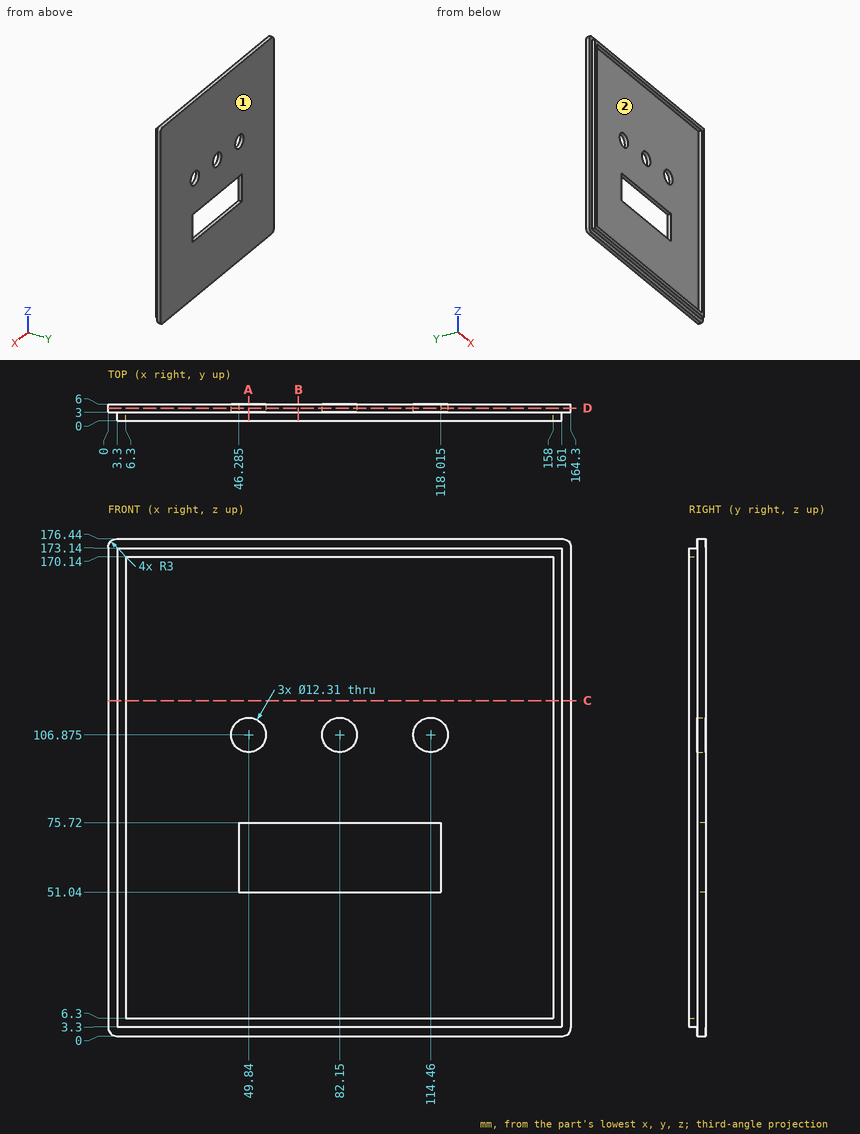
Job drawing, mm, ordinate dimensions from the low corner. One solid piece. Round coordinates to 2 decimals unless told otherwise and drop trailing zeros. Write each loop counter-clockwise with the first axis right and the second up, starting at its lowest first coordinate (ties: lowest second). Pieces come first, ordered by that corner, then holes. Notation, with made-up numbers: M 81.25,36 L 93.25,36 A31 ccw 93.25,63 Z; hole C 9,62 d2. An arc over 180 degrees is marked long. Return JSON: item names as keys, results as strings. Group by question number.
(1) Saw through at A-A on x = 49.84. Write the cut outline in (y, z).
(2) Drill centre lines: probe 1 along Z at (x, y) = (49.84, 4.2); probe 2 along X at (y, z) = (2.7, 29); probe 3 along Z at (x, y) = (57, 4.5). Where is each one in solid material? Low to high.
(3) Saw through at B-B on x = 67.5. Write the cut outline in (y, z), then the cut area to 3 significant figures.
(4) Saw through at C-C on z = 119. Write the cut outline in (x, y), then the cut area to 3 significant figures.
(5) Two-plate mould, pull along Z, no slides. Class the marked faces 1 and 2: +Z half, -Z half, draft (parallel to the pull), parting line (faces both ways), or undercut.
(6) Saw through at D-D on y = 4.5. Write the cut outline in (x, z) (3 decimals), then the cut area to 3 significant figures.
(7) Pin check, flat tips, straight feed: pin 1 Ø8 at (x, z) = (129.5, 55) entering from -Y; pin 2 Ø3.5 at (x, y) = (61, 1) entering from +Z; pin 3 Ø1 at (x, y) = (32, 1) entering from -Z. Stop position of each tip, or through.
Returned:
{
 "1": {"outline": "M 0,3.3 L 3,3.3 L 3,0 L 6,0 L 6,51.04 L 3,51.04 L 3,6.3 L 0,6.3 Z; M 0,170.14 L 3,170.14 L 3,113.03 L 6,113.03 L 6,176.44 L 3,176.44 L 3,173.14 L 0,173.14 Z; M 3,75.72 L 6,75.72 L 6,100.72 L 3,100.72 Z"},
 "2": {"probe 1": "0 to 51.04, 75.72 to 100.72, 113.03 to 176.44", "probe 2": "3.3 to 6.3, 158 to 161", "probe 3": "0 to 51.04, 75.72 to 176.44"},
 "3": {"outline": "M 0,3.3 L 3,3.3 L 3,0 L 6,0 L 6,51.04 L 3,51.04 L 3,6.3 L 0,6.3 Z; M 0,170.14 L 3,170.14 L 3,75.72 L 6,75.72 L 6,176.44 L 3,176.44 L 3,173.14 L 0,173.14 Z", "area": "473 mm²"},
 "4": {"outline": "M 0,3 L 3.3,3 L 3.3,0 L 6.3,0 L 6.3,3 L 158,3 L 158,0 L 161,0 L 161,3 L 164.3,3 L 164.3,6 L 0,6 Z", "area": "511 mm²"},
 "5": {"face 1": "draft", "face 2": "undercut"},
 "6": {"outline": "M 0,3 A3 ccw 3,0 L 161.3,0 A3 ccw 164.3,3 L 164.3,173.44 A3 ccw 161.3,176.44 L 3,176.44 A3 ccw 0,173.44 Z; hole C 49.84,106.875 d12.31; hole M 46.285,51.04 L 118.015,51.04 L 118.015,75.72 L 46.285,75.72 Z; hole C 82.15,106.875 d12.31; hole C 114.46,106.875 d12.31", "area": "26,900 mm²"},
 "7": {"pin 1": "y = 3", "pin 2": "z = 173.14", "pin 3": "z = 3.3"}
}
